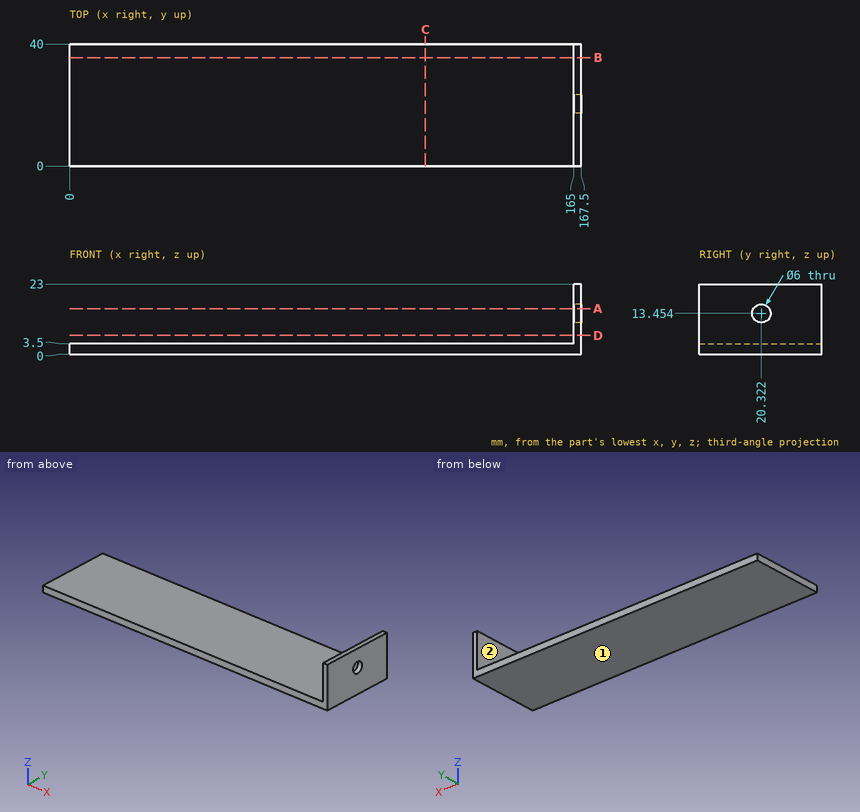
Input: dimensioned drawing with shaded views. Units: mm. Origin: part minimum x, y, z. A direction names the side the tool comes from. Give positions to 0.01 mm unless a question says otherwise; leave off trailing zeros. Order: outer loops, then holes, each group sorted by start corner. A loop starts at its lowest first (then second) coordinate and runs counter-clockwise, first axis right, second up. Notation, with made-up numbers: (-32.5, 34) -> (-13.5, 34) arc R21 cw to (-13.5, 44) -> close; hole circle Ø2 at (3, 87.5). An arc over 180 degrees is marked (long way). Answer as a JSON object with one key per item and string values.
Q1. First-contact query: pin 1 (20 mm diameter, centred on x = 98, y = 23.5, fed in from +Z); pin 2 (3 mm diameter, centred on y = 6.5, z = 13.5, fed in from -X). Flat tips, straight axial feed; report the tip coordinate or a pass-through.
Entries:
{"pin 1": "stops at z = 3.5", "pin 2": "stops at x = 165"}
Q2. Section B-B (y = 35.5). Output: boundary loops of the cut face in (x, z).
Entries:
{"outline": "(0, 0) -> (167.5, 0) -> (167.5, 23) -> (165, 23) -> (165, 3.5) -> (0, 3.5) -> close"}
Q3. Section D-D (z = 6.25). Output: boundary loops of the cut face in (x, y), plus the area to 3 significant figures.
Entries:
{"outline": "(165, 0) -> (167.5, 0) -> (167.5, 40) -> (165, 40) -> close", "area": "100 mm^2"}
Q4. Access query for the marked faces 1 and 2. Directions: +Z, -Z, +X, -X, +Y, -Y. A direction counts if a zero-diameter tool reaches every point of the face in a straight line with its end or side. Return the directions, or none.
Entries:
{"face 1": "-Z, +X, -X, +Y, -Y", "face 2": "+Z, -X, +Y, -Y"}
Q5. Material intervals for probe 1 along X at (y, z) = (7.5, 15.75); probe 2 along Z at (x, y) = (100, 18), sorted ascending.
Entries:
{"probe 1": "x = 165 to 167.5", "probe 2": "z = 0 to 3.5"}
Q6. Section A-A (z = 15). Output: boundary loops of the cut face in (x, y).
Entries:
{"outline": "(165, 0) -> (167.5, 0) -> (167.5, 17.75) -> (165, 17.75) -> close; (165, 22.89) -> (167.5, 22.89) -> (167.5, 40) -> (165, 40) -> close"}
Q7. Section C-C (x = 116.5). Output: boundary loops of the cut face in (y, z).
Entries:
{"outline": "(0, 0) -> (40, 0) -> (40, 3.5) -> (0, 3.5) -> close"}
